from build123d import *

# Parameters (mm, degrees)
SKETCH1_W           = 130
SKETCH1_H           = 126
BOSS_EXTRUDE1_DEPTH = 120
SKETCH3_W           = 120
SKETCH3_H           = 110
CUT_EXTRUDE3_DEPTH  = 121
SKETCH2_R           = 11
SKETCH2_R_2         = 3.55
SKETCH2_R_3         = 6.1
SKETCH2_R_4         = 3.4
SKETCH2_R_5         = 2.476
CUT_EXTRUDE4_DEPTH  = 5
SKETCH6_R           = 51.5
SKETCH6_R_2         = 2.05
CUT_EXTRUDE5_DEPTH  = 5
SKETCH7_W           = 120
SKETCH7_H           = 110
SKETCH7_W_2         = 108
SKETCH7_H_2         = 98
BOSS_EXTRUDE2_DEPTH = 6
SKETCH8_W           = 112
SKETCH8_H           = 102
SKETCH8_W_2         = 108
SKETCH8_H_2         = 98
BOSS_EXTRUDE3_DEPTH = 3
SKETCH9_R           = 3
CUT_EXTRUDE6_DEPTH  = 4
CHAMFER2_SIZE       = 6
SKETCH10_R          = 1.75
SKETCH10_W          = 32.45
SKETCH10_H          = 20.574
CUT_EXTRUDE10_DEPTH = 10
FILLET4_R           = 3
SKETCH16_R          = 25.5
CUT_EXTRUDE9_DEPTH  = 2
SKETCH18_R          = 27.25
SKETCH18_R_2        = 25.25
BOSS_EXTRUDE4_DEPTH = 28.16
SKETCH19_R          = 27.25
BOSS_EXTRUDE5_DEPTH = 2
SKETCH20_R          = 3.55
SKETCH20_R_2        = 11
CUT_EXTRUDE11_DEPTH = 51
SKETCH21_R          = 25.5
CUT_EXTRUDE12_DEPTH = 31.16


with BuildPart() as part:
    # Sketch1 → Boss-Extrude1 (new body)
    with BuildSketch(Plane.XY):
        Rectangle(SKETCH1_W, SKETCH1_H)
    extrude(amount=BOSS_EXTRUDE1_DEPTH)

    # Sketch3 → Cut-Extrude3 (cut)
    with BuildSketch(Plane(origin=(0, 63, 0), x_dir=(1, 0, 0), z_dir=(0, 1, 0))):
        with Locations((0, -60)):
            Rectangle(SKETCH3_W, SKETCH3_H)
    extrude(amount=-CUT_EXTRUDE3_DEPTH, mode=Mode.SUBTRACT)

    # Sketch2 → Cut-Extrude4 (cut)
    with BuildSketch(Plane.XY.offset(120)):
        with Locations((32, 31)):
            Circle(SKETCH2_R)
        with Locations((32, 49.7)):
            Circle(SKETCH2_R_2)
        with Locations((-46.2, -6.9)):
            Circle(SKETCH2_R_3)
        with Locations((-29.08, -5.56)):
            Circle(SKETCH2_R_4)
        with Locations((-29.08, 12.19)):
            Circle(SKETCH2_R_4)
        with Locations((-29.08, -23.31)):
            Circle(SKETCH2_R_4)
        with Locations((-6.1, -22.81)):
            Circle(SKETCH2_R_5)
        with Locations((-6.1, -5.31)):
            Circle(SKETCH2_R_5)
        with Locations((-6.1, 12.19)):
            Circle(SKETCH2_R_5)
        with Locations((32, -49.7)):
            Circle(SKETCH2_R_2)
        with Locations((32, 12.3)):
            Circle(SKETCH2_R_2)
        with Locations((32, -31)):
            Circle(SKETCH2_R)
        with Locations((32, -12.3)):
            Circle(SKETCH2_R_2)
    extrude(amount=-CUT_EXTRUDE4_DEPTH, mode=Mode.SUBTRACT)

    # Sketch6 → Cut-Extrude5 (cut)
    with BuildSketch(Plane(origin=(0, 0, 0), x_dir=(-1, 0, 0), z_dir=(0, 0, -1))):
        with Locations((0, -1.25)):
            Circle(SKETCH6_R)
        with Locations((40.128309832, -41.378309832)):
            Circle(SKETCH6_R_2)
        with Locations((-40.128309832, -41.378309832)):
            Circle(SKETCH6_R_2)
        with Locations((40.128309832, 38.878309832)):
            Circle(SKETCH6_R_2)
        with Locations((-40.128309832, 38.878309832)):
            Circle(SKETCH6_R_2)
    extrude(amount=-CUT_EXTRUDE5_DEPTH, mode=Mode.SUBTRACT)

    # Sketch7 → Boss-Extrude2 (add)
    with BuildSketch(Plane(origin=(0, 63, 0), x_dir=(1, 0, 0), z_dir=(0, 1, 0))):
        with Locations((0, -60)):
            Rectangle(SKETCH7_W, SKETCH7_H)
        with Locations((0, -60)):
            Rectangle(SKETCH7_W_2, SKETCH7_H_2, mode=Mode.SUBTRACT)
    extrude(amount=-BOSS_EXTRUDE2_DEPTH)

    # Sketch8 → Boss-Extrude3 (add)
    with BuildSketch(Plane(origin=(0, 63, 0), x_dir=(1, 0, 0), z_dir=(0, 1, 0))):
        with Locations((0, -60)):
            Rectangle(SKETCH8_W, SKETCH8_H)
        with Locations((0, -60)):
            Rectangle(SKETCH8_W_2, SKETCH8_H_2, mode=Mode.SUBTRACT)
    extrude(amount=BOSS_EXTRUDE3_DEPTH)

    # Sketch9 → Cut-Extrude6 (cut)
    with BuildSketch(Plane(origin=(0, 63, 0), x_dir=(1, 0, 0), z_dir=(0, 1, 0))):
        with Locations(Location((-60, -5, 0), (0, 0, 180))):
            Circle(SKETCH9_R)
        with Locations(Location((-60, -115, 0), (0, 0, 180))):
            Circle(SKETCH9_R)
        with Locations(Location((60, -115, 0), (0, 0, 180))):
            Circle(SKETCH9_R)
        with Locations(Location((60, -5, 0), (0, 0, 180))):
            Circle(SKETCH9_R)
    extrude(amount=-CUT_EXTRUDE6_DEPTH, mode=Mode.SUBTRACT)

    # Chamfer2
    chamfer2_edges = [part.edges().sort_by_distance(p)[0] for p in [
        (0, 57, 11),
        (-54, 57, 60),
        (0, 57, 109),
        (54, 57, 60),
    ]]
    chamfer(chamfer2_edges, length=CHAMFER2_SIZE - 0.0001)  # a hair under: the kernel refuses the full size

    # Sketch10 → Cut-Extrude10 (cut)
    with BuildSketch(Plane.ZY.offset(65)):
        with Locations((63.241, -24.894)):
            Circle(SKETCH10_R)
        with Locations((108.25, -24.894)):
            Circle(SKETCH10_R)
        with Locations((108.25, -49.597)):
            Circle(SKETCH10_R)
        with Locations((63.241, -49.597)):
            Circle(SKETCH10_R)
        with Locations((77.14, 42.7)):
            Circle(SKETCH10_R)
        with Locations((108.25, 42.7)):
            Circle(SKETCH10_R)
        with Locations((108.25, 19.53)):
            Circle(SKETCH10_R)
        with Locations((77.14, 19.53)):
            Circle(SKETCH10_R)
        with Locations((85.7455, -37.2455)):
            Rectangle(SKETCH10_W, SKETCH10_H)
        Polygon((86.345, 24.215), (83.195, 24.215), (83.195, 38.015), (102.195, 38.015), (102.195, 24.215), (99.045, 24.215), (99.045, 21.215), (86.345, 21.215), align=None)
    extrude(amount=-CUT_EXTRUDE10_DEPTH, mode=Mode.SUBTRACT)

    # Fillet4
    fillet4_edges = [part.edges().sort_by_distance(p)[0] for p in [
        (65, 0, 120),
        (-65, 0, 120),
        (65, 0, 0),
        (-65, 0, 0),
    ]]
    fillet(fillet4_edges, radius=FILLET4_R)

    # Sketch16 → Cut-Extrude9 (cut)
    with BuildSketch(Plane.XY.offset(120)):
        with Locations((32, 31)):
            Circle(SKETCH16_R)
        with Locations((32, -31)):
            Circle(SKETCH16_R)
    extrude(amount=-CUT_EXTRUDE9_DEPTH, mode=Mode.SUBTRACT)

    # Sketch18 → Boss-Extrude4 (add)
    # profile 1 of 2: a face of its own
    with BuildSketch(Plane(origin=(0, 0, 115), x_dir=(-1, 0, 0), z_dir=(0, 0, -1))):
        with Locations((-32, -31)):
            Circle(SKETCH18_R)
        with Locations((-32, -31)):
            Circle(SKETCH18_R_2, mode=Mode.SUBTRACT)
    # profile 2 of 2: a face of its own
    with BuildSketch(Plane(origin=(0, 0, 115), x_dir=(-1, 0, 0), z_dir=(0, 0, -1))):
        with BuildLine():
            Line((-40.158584436, 57), (-23.841415564, 57))
            ThreePointArc((-23.841415564, 57), (-32, 3.75), (-40.158584436, 57))
        make_face()
        with Locations((-32, 31)):
            Circle(SKETCH18_R_2, mode=Mode.SUBTRACT)
    extrude(amount=BOSS_EXTRUDE4_DEPTH)

    # Sketch19 → Boss-Extrude5 (add)
    with BuildSketch(Plane(origin=(0, 0, 86.84), x_dir=(-1, 0, 0), z_dir=(0, 0, -1))):
        with Locations((-32, -31)):
            Circle(SKETCH19_R)
        with BuildLine():
            Line((-40.158584436, 57), (-23.841415564, 57))
            ThreePointArc((-23.841415564, 57), (-32, 3.75), (-40.158584436, 57))
        make_face()
    extrude(amount=BOSS_EXTRUDE5_DEPTH)

    # Sketch20 → Cut-Extrude11 (cut)
    with BuildSketch(Plane.XY.offset(118)):
        with Locations((32, 49.7)):
            Circle(SKETCH20_R)
        with Locations((32, 31)):
            Circle(SKETCH20_R_2)
        with Locations((32, 12.3)):
            Circle(SKETCH20_R)
        with Locations((32, -31)):
            Circle(SKETCH20_R_2)
        with Locations((32, -12.3)):
            Circle(SKETCH20_R)
        with Locations((32, -49.7)):
            Circle(SKETCH20_R)
    extrude(amount=-CUT_EXTRUDE11_DEPTH, mode=Mode.SUBTRACT)

    # Sketch21 → Cut-Extrude12 (cut)
    with BuildSketch(Plane.XY.offset(118)):
        with Locations((32, 31)):
            Circle(SKETCH21_R)
        with Locations((32, -31)):
            Circle(SKETCH21_R)
    extrude(amount=-CUT_EXTRUDE12_DEPTH, mode=Mode.SUBTRACT)


solid = part.part
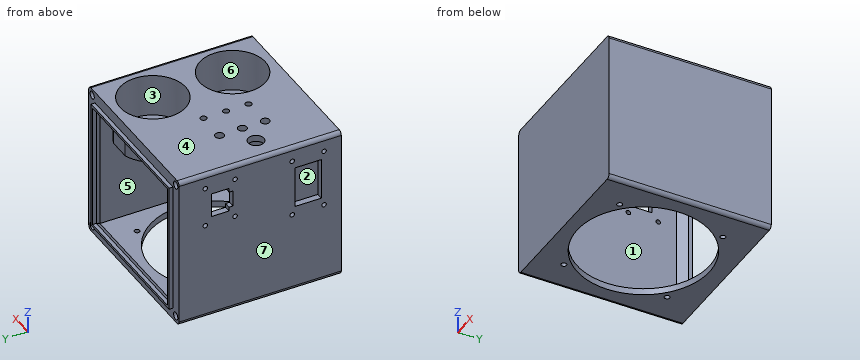
Part model, mm, in its own coordinate system. Face numbers are marked on the shaded views. A direction names the side the tool comes from. Give positions to 0.01 mm unless a question says otherwise; leave off trailing zeros. Write each question's results on one line, items separated by ' | '. Start each with the question number.
Q1. Band-saw the part on B-B on y = -34. Count the separate pieces of the cut face and the enclosed holes in it, plus the area to 3 significant figures.
Q2. Pin check, flat tips, straight feed: P1, Ø1.5, axis at x = -63, y = 22.5, coming from the -Z side; P2, Ø5, axis at x = -7, z = 73.5, coming from the +Y side; P3, Ø5.5, axis at x = -29.08, y = 12.19, coming from the -Z side; P4, Ø1.5, axis at y = 64.5, z = 46, coming from the +X side. Stop position of each tip, or through.
Q3. Which spindle directions (+Z, -Z, +X, -X, +Y, -Y) get a long thin tool onto all of the face, cutting with end or side? Do the marked faces 5, 6 and 7. Say none if no direction does.
Q4. Wall check: L1, parallel to Y at x = -62.65, z = 77.14; L2, parallel to Y at x = -29.08, z = 116.6; L3, parallel to Z at x = 24, y = -56.5. Give the ranges that are in metal, low to high.
Q5. Pull direction Z, two halves, no side cores. Call the marked faces 1, 2, 3 and 4: +Z half, -Z half, draft (parallel to the pull), parting line (faces both ways), or undercut.
Results are:
1) separate pieces: 3 | enclosed holes: 0 | area: 1,740 mm²
2) P1: stops at z = 0.01 | P2: stops at y = -58 | P3: passes through | P4: stops at x = 56
3) face 5: none | face 6: +Z | face 7: +Z, -Z, -X, +Y, -Y
4) L1: y = -63 to -47.53, -26.96 to 17.78, 21.28 to 40.95, 44.45 to 63 | L2: y = -63 to -26.71, -19.91 to -8.96, -2.16 to 8.79, 15.59 to 63 | L3: z = 0 to 5, 84.84 to 120
5) face 1: undercut | face 2: undercut | face 3: draft | face 4: +Z half
